Design review of the part built by this model. Coordinates are the model's own, in mm. Coordinates: 2 decimals unless noted, no trailing zeros. Loops run counter-clockwise (first coordinate to the right, second up) from the corner with the lowest first, then second, coordinate; pieces in that order, holes last. Notation, with made-up numbers: M 75,-0.75 L 89,-0.75 A29 cw 89,24.25 Z; hole C 8,63.5 d9. An arc over 180 degrees is marked long. One line per item, written item: value.
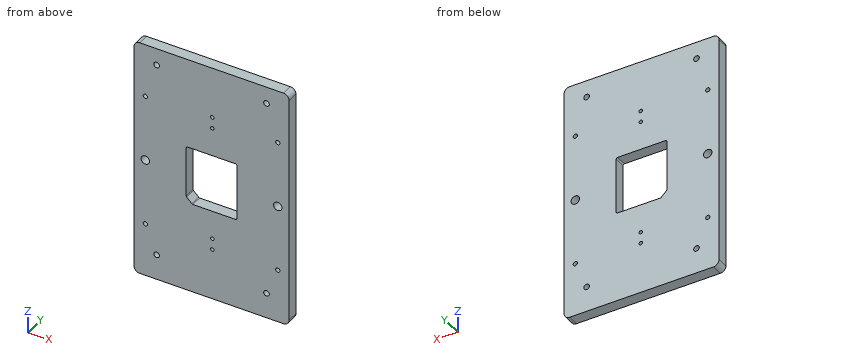
```python
from build123d import *

# Parameters (mm, degrees)
SALIENTE_EXTRUIR1_DEPTH = 8
CROQUIS2_R              = 2
CROQUIS2_R_2            = 1.5
CROQUIS2_R_3            = 3
CORTAR_EXTRUIR1_DEPTH   = 18
CROQUIS3_W              = 36
CROQUIS3_H              = 41
CORTAR_EXTRUIR2_DEPTH   = 8
CROQUIS4_W              = 50
CROQUIS4_H              = 90
CORTAR_EXTRUIR3_DEPTH   = 8
CROQUIS5_W              = 59.93105858
CROQUIS5_H              = 100.56613239
SALIENTE_EXTRUIR2_DEPTH = 8
CROQUIS7_W              = 94.273148937
CROQUIS7_H              = 8.636825756
SALIENTE_EXTRUIR3_DEPTH = 8
CROQUIS8_R              = 2
CORTAR_EXTRUIR4_DEPTH   = 102.557865279
CROQUIS9_R              = 1.25
CORTAR_EXTRUIR5_DEPTH   = 8


with BuildPart() as part:
    # Croquis1 → Saliente-Extruir1 (new body)
    with BuildSketch(Plane(origin=(0, 0, 0), x_dir=(1, 0, 0), z_dir=(0, 1, 0))):
        with BuildLine():
            Line((-51, 85), (51, 85))
            ThreePointArc((51, 85), (53.828427125, 83.828427125), (55, 81))
            Line((55, 81), (55, -81))
            ThreePointArc((55, -81), (53.828427125, -83.828427125), (51, -85))
            Line((51, -85), (-51, -85))
            ThreePointArc((-51, -85), (-53.828427125, -83.828427125), (-55, -81))
            Line((-55, -81), (-55, 81))
            ThreePointArc((-55, 81), (-53.828427125, 83.828427125), (-51, 85))
        make_face()
    extrude(amount=SALIENTE_EXTRUIR1_DEPTH)

    # Croquis2 → Cortar-Extruir1 (cut)
    with BuildSketch(Plane(origin=(0, 8, 0), x_dir=(1, 0, 0), z_dir=(0, 1, 0))):
        with Locations(Location((-39, 73, 0), (0, 0, 270))):
            Circle(CROQUIS2_R)
        with Locations(Location((-47, 47, 0), (0, 0, 270))):
            Circle(CROQUIS2_R_2)
        with Locations(Location((47, 47, 0), (0, 0, 270))):
            Circle(CROQUIS2_R_2)
        with Locations(Location((39, 73, 0), (0, 0, 270))):
            Circle(CROQUIS2_R)
        with Locations(Location((39, -73, 0), (0, 0, 270))):
            Circle(CROQUIS2_R)
        with Locations(Location((47, -47, 0), (0, 0, 270))):
            Circle(CROQUIS2_R_2)
        with Locations(Location((-47, -47, 0), (0, 0, 270))):
            Circle(CROQUIS2_R_2)
        with Locations(Location((-39, -73, 0), (0, 0, 270))):
            Circle(CROQUIS2_R)
        with Locations(Location((-47, 0, 0), (0, 0, 270))):
            Circle(CROQUIS2_R_3)
        with Locations(Location((47, 0, 0), (0, 0, 270))):
            Circle(CROQUIS2_R_3)
    extrude(amount=-CORTAR_EXTRUIR1_DEPTH, mode=Mode.SUBTRACT)

    # Croquis3 → Cortar-Extruir2 (cut)
    with BuildSketch(Plane(origin=(0, 8, 0), x_dir=(1, 0, 0), z_dir=(0, 1, 0))):
        Rectangle(CROQUIS3_W, CROQUIS3_H)
    extrude(amount=-CORTAR_EXTRUIR2_DEPTH, mode=Mode.SUBTRACT)

    # Croquis4 → Cortar-Extruir3 (cut)
    with BuildSketch(Plane.XZ):
        Rectangle(CROQUIS4_W, CROQUIS4_H)
    extrude(amount=-CORTAR_EXTRUIR3_DEPTH, mode=Mode.SUBTRACT)

    # Croquis5 → Saliente-Extruir2 (add)
    with BuildSketch(Plane.XZ):
        with Locations((0.580457048, 0.547604551)):
            Rectangle(CROQUIS5_W, CROQUIS5_H)
        with BuildLine():
            Line((-13.343145751, -20.5), (17, -20.5))
            ThreePointArc((17, -20.5), (17.707106781, -20.207106781), (18, -19.5))
            Line((18, -19.5), (18, 19.5))
            ThreePointArc((18, 19.5), (17.707106781, 20.207106781), (17, 20.5))
            Line((17, 20.5), (-17, 20.5))
            ThreePointArc((-17, 20.5), (-17.707106781, 20.207106781), (-18, 19.5))
            Line((-18, 19.5), (-18, -15.843145751))
            ThreePointArc((-18, -15.843145751), (-17.923879533, -16.225829183), (-17.707106781, -16.550252532))
            Line((-17.707106781, -16.550252532), (-14.050252532, -20.207106781))
            ThreePointArc((-14.050252532, -20.207106781), (-13.725829183, -20.423879533), (-13.343145751, -20.5))
        make_face(mode=Mode.SUBTRACT)
    extrude(amount=-SALIENTE_EXTRUIR2_DEPTH)

    # Croquis7 → Saliente-Extruir3 (add)
    with BuildSketch(Plane(origin=(0, 8, 0), x_dir=(1, 0, 0), z_dir=(0, 1, 0))):
        with Locations((1.18677705, 71.991192559)):
            Rectangle(CROQUIS7_W, CROQUIS7_H)
    extrude(amount=-SALIENTE_EXTRUIR3_DEPTH)

    # Croquis8 → Cortar-Extruir4 (cut, through all)
    with BuildSketch(Plane(origin=(0, 8, 0), x_dir=(1, 0, 0), z_dir=(0, 1, 0))):
        with Locations(Location((-39, 67, 0), (0, 0, 270))):
            Circle(CROQUIS8_R)
        with Locations(Location((39, 67, 0), (0, 0, 270))):
            Circle(CROQUIS8_R)
    extrude(amount=-CORTAR_EXTRUIR4_DEPTH, mode=Mode.SUBTRACT)

    # Croquis9 → Cortar-Extruir5 (cut)
    with BuildSketch(Plane.XZ):
        with Locations(Location((0.547678372, 40.686961559, 0), (0, 0, 270))):
            Circle(CROQUIS9_R)
        with Locations(Location((0.547678372, 48.686961559, 0), (0, 0, 270))):
            Circle(CROQUIS9_R)
        with Locations(Location((0.547678372, -48.686961559, 0), (0, 0, 90))):
            Circle(CROQUIS9_R)
        with Locations(Location((0.547678372, -40.686961559, 0), (0, 0, 90))):
            Circle(CROQUIS9_R)
    extrude(amount=-CORTAR_EXTRUIR5_DEPTH, mode=Mode.SUBTRACT)


solid = part.part
```
(1) We need section B-B on z = 0. State the section outline as (x, y) points, then the cut area to 3 significant figures.
Reply:
outline: M -55,0 L -50,0 L -50,8 L -55,8 Z; M -44,0 L -18,0 L -18,8 L -44,8 Z; M 18,0 L 44,0 L 44,8 L 18,8 Z; M 50,0 L 55,0 L 55,8 L 50,8 Z
area: 496 mm2
(2) We need section C-C on y = 5.5. State how many separate pieces and enclosed holes the cut face has, then the cut area to 3 significant figures.
Reply:
separate pieces: 1
enclosed holes: 15
area: 17,100 mm2
(3) We need section D-D on x = -39. State the section outline as (y, z) points.
Reply:
outline: M 0,-85 L 8,-85 L 8,-69 L 0,-69 Z; M 0,-65 L 8,-65 L 8,71 L 0,71 Z; M 0,75 L 8,75 L 8,85 L 0,85 Z
(4) To check wall thickness, follow line 1 along X through (y, z) = (4.75, -47); line 2 along X through (y, z) = (6.75, -67); line 3 along Z through (x, y) = (-2, 5). State the ranges of each line that lie inside material, in increasing order. Write a range as [from, to].
Reply:
line 1: x = [-55, -48.5], [-45.5, 45.5], [48.5, 55]
line 2: x = [-55, -41], [-37, 37], [41, 55]
line 3: z = [-85, -20.5], [20.5, 85]
(5) We need section A-A on x = -4.5. State the section outline as (y, z) points.
Reply:
outline: M 0,-85 L 8,-85 L 8,-20.5 L 0,-20.5 Z; M 0,20.5 L 8,20.5 L 8,85 L 0,85 Z
(6) Insertion check: pin 1 (3.5 mm diameter, centred on x = 39, z = -67, fed in from +Y). The pin has a flat end and moves straight along its axis. Give the tip position at first contact, or say it passes through.
Reply:
pin 1: passes through
